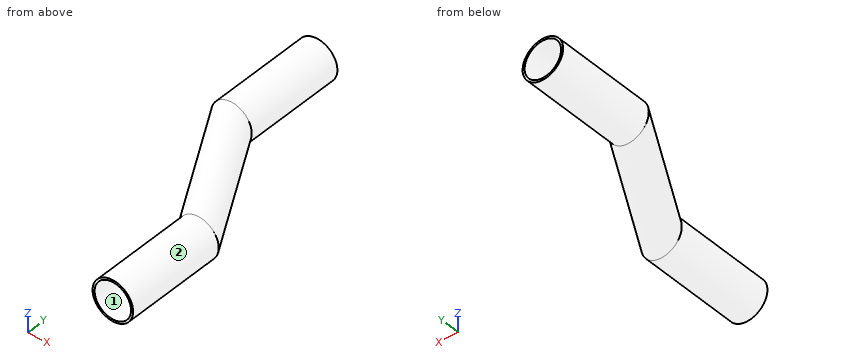
```python
from build123d import *

# Parameters (mm, degrees)
SKETCH1_R           = 10
SKETCH1_R_2         = 9
BOSS_EXTRUDE1_DEPTH = 50
SKETCH2_R           = 10
SKETCH2_R_2         = 9
SKETCH4_R           = 10
SKETCH4_R_2         = 9


with BuildPart() as part:
    # Sketch1 → Boss-Extrude1 (new body)
    with BuildSketch(Plane(origin=(0, 0, 0), x_dir=(1, 0, 0), z_dir=(0, 1, 0))):
        with Locations(Location((0, 0, 0), (0, 0, 270))):
            Circle(SKETCH1_R)
        with Locations(Location((0, 0, 0), (0, 0, 270))):
            Circle(SKETCH1_R_2, mode=Mode.SUBTRACT)
    extrude(amount=BOSS_EXTRUDE1_DEPTH)

    # Sweep1: sweep along a path in Sketch3
    with BuildLine(Plane.XY) as sweep1_path:
        Line((0, 0), (35, -60.621778265))
    # Sketch2 → Sweep1 (sweep)
    with BuildSketch(Plane.XZ):
        Circle(SKETCH2_R)
        Circle(SKETCH2_R_2, mode=Mode.SUBTRACT)
    sweep(path=sweep1_path.line)

    # Sweep2: sweep along a path in Sketch5
    with BuildLine(Plane.XY) as sweep2_path:
        Line((35, -60.621778265), (35, -110.621778265))
    # Sketch4 → Sweep2 (sweep)
    with BuildSketch(Plane.XZ.offset(60.621778265)):
        with Locations((35, 0)):
            Circle(SKETCH4_R)
        with Locations((35, 0)):
            Circle(SKETCH4_R_2, mode=Mode.SUBTRACT)
    sweep(path=sweep2_path.line)


solid = part.part
```
The listing builds one solid part. Answer for the finished solid, in the listing's coordinates (mm). Face numbers are marked on the shaded views. Round coordinates to 2 decimals unless told otherwise and drop trailing zeros. Loops run counter-clockwise (first coordinate to the right, second up) from the corner with the lowest first, then second, coordinate; pieces in that order, holes last.
Q1. For a pull along Z with two mould halves and no side action, classify the marked faces 1 and 2 as released by +Z, released by -Z, zero draft, split by the parting line, or undercut.
Q2. Section A-A, the plane y = -86.5 is taken. Determine the outline of the cut face in (x, z), then the cut area to 3 significant figures.
Q3. Find the intervals of material crossed by line 1 (Z direction, x = 0, y = 36); line 2 (Z direction, x = 30, y = -77.5), in increasing order.
Q4. Given pin 1 Ø10 at (y, z) = (-67, 7) entering from -X; pin 2 Ø5 at (x, z) = (36.5, -3) entering from +Y; pin 3 Ø6 at (y, z) = (21.5, 6.5) entering from +X, each flat-ended and moving along its own axis, determine where each tip first touches the part or whether it passes through.
Completed:
1. face 1: undercut
1. face 2: split by the parting line
2. outline: circle Ø20 at (35, 0); hole circle Ø18 at (35, 0)
2. area: 59.7 mm2
3. line 1: z = -10 to -9, 9 to 10
3. line 2: z = -8.66 to -7.48, 7.48 to 8.66
4. pin 1: stops at x = 25.2
4. pin 2: stops at y = -42.2
4. pin 3: stops at x = 9.37
